Verification items for this drawing (mm, ordinates from the low corner). A direction names the side the tool comes from. Coordinates: 2 decimals unless noted, no trailing zeros. Order: outer loops, then holes, each group sorted by start corner. A loop starts at its lowest first (then second) coordinate and runs counter-clockwise, first axis right, second up.
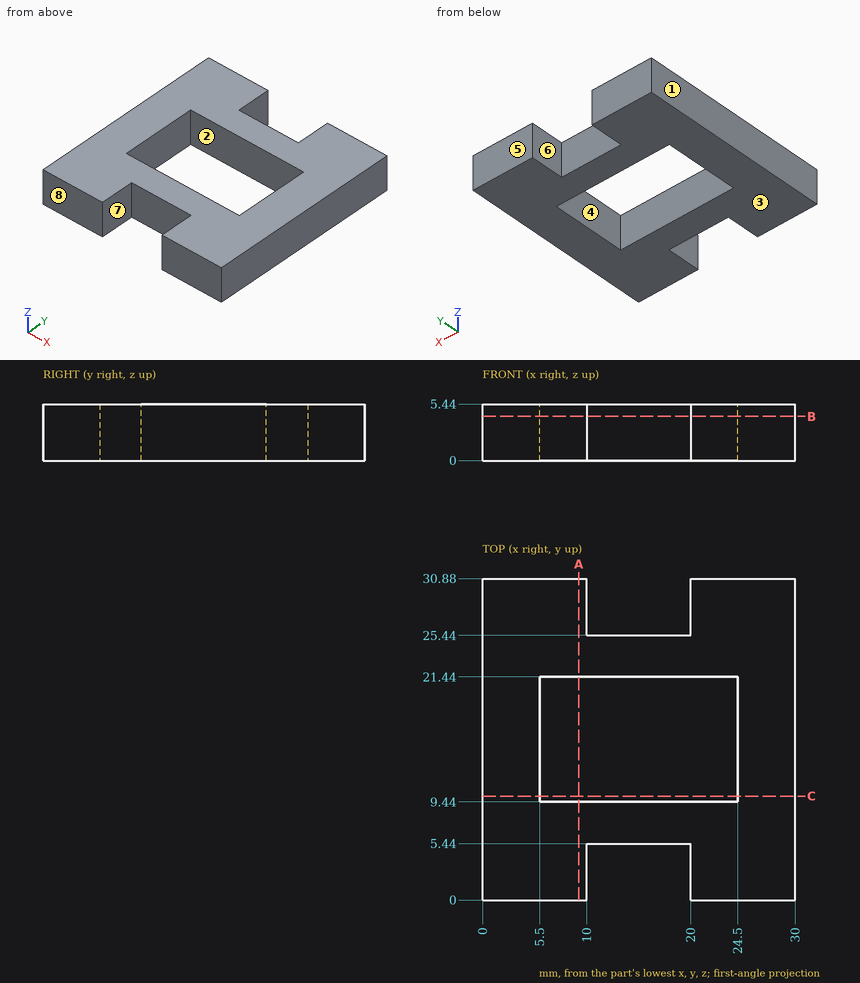
(1) Cross-section at A-A (x = 9.25). Enter the section's corners in (y, z).
Filled in:
outline: (0, 0) - (9.44, 0) - (9.44, 5.44) - (0, 5.44) - close; (21.44, 0) - (30.88, 0) - (30.88, 5.44) - (21.44, 5.44) - close
(2) Release check for a two-part mould opening along X. For the marked faces 1, 2 and 3 record: +X half, -X half, draft (parallel to the pull), parting line (faces both ways), or undercut.
Filled in:
face 1: -X half
face 2: undercut
face 3: draft
(3) Thickness scan on probe 1 along X at (y, z) = (29.5, 5.2); probe 2 along X at (y, z) = (19.5, 3.25); probe 3 along Y at (x, z) = (8.25, 0.7). Record the ranges inside material, lowest first.
Filled in:
probe 1: x = 0 to 10, 20 to 30
probe 2: x = 0 to 5.5, 24.5 to 30
probe 3: y = 0 to 9.44, 21.44 to 30.88
(4) Cross-section at C-C (y = 10). Enter the section's corners in (x, z), and give its area (3 significant figures).
Filled in:
outline: (0, 0) - (5.5, 0) - (5.5, 5.44) - (0, 5.44) - close; (24.5, 0) - (30, 0) - (30, 5.44) - (24.5, 5.44) - close
area: 59.8 mm2
(5) Cross-section at B-B (z = 4.25). Enter the section's corners in (x, y).
Filled in:
outline: (0, 0) - (10, 0) - (10, 5.44) - (20, 5.44) - (20, 0) - (30, 0) - (30, 30.88) - (20, 30.88) - (20, 25.44) - (10, 25.44) - (10, 30.88) - (0, 30.88) - close; hole (5.5, 9.44) - (24.5, 9.44) - (24.5, 21.44) - (5.5, 21.44) - close
(6) Tool access check on the marked faces 4, 5, 6, 7 and 8. Record the directions out of +Z, -Z, +X, -X, +Y, -Y that give a thin tool (end or side, any length) a straight path to the whole face; none if there is none.
Filled in:
face 4: +Z, -Z
face 5: +Z, -Z, +X, -X, +Y
face 6: +Z, -Z, +Y
face 7: +Z, -Z, -Y
face 8: +Z, -Z, +X, -X, -Y
(7) Go/stop test with flat-tipped pins: P1, Ø2, axis at x = 18.5, z = 3.5, coming from the +Y side; P2, Ø2.5, axis at x = 14.5, z = 3, coming from the -Y side. Record where each tip stops, or that it passes through.
Filled in:
P1: stops at y = 25.44
P2: stops at y = 5.44
